```python
from build123d import *

# Parameters (mm, degrees)
F1_DEPTH = 50
F2_R     = 3
F3_DEPTH = 10


with BuildPart() as f1:
    # F0 (on Front) → F1 (new body)
    with BuildSketch(Plane.XZ):
        Polygon((-25, 2.796772), (-25, -15.488228), (25, -15.488228), (0, 2.796772), align=None)
    extrude(amount=F1_DEPTH)

    # F2 (on face) → F3 (join)
    with BuildSketch(Plane.XY.offset(2.796772)):
        with Locations((-13.586, -13.45)):
            Circle(F2_R)
        with Locations((-13.156, -36.55)):
            Circle(F2_R)
    extrude(amount=F3_DEPTH)


with BuildPart() as f4_1:
    # F4: instance of F1
    add(f1.part.mirror(Plane.YZ))


solid = f4_1.part
```
Design review of the part built by this model. Coordinates are the model's own, in mm. A direction names the side the tool comes from. Coordinates: 2 decimals unless noted, no trailing zeros. Loops run counter-clockwise (first coordinate to the right, second up) from the corner with the lowest first, then second, coordinate; pieces in that order, holes last. Notation, with made-up numbers: (-22, 80.25) -> (11, 80.25) arc R26 cw to (11, 111.25) -> close; hole circle Ø11 at (18.25, 10.25). An arc over 180 degrees is marked (long way). Answer as a JSON object with one key per item and string values.
Q1. Tool access review of faces 1 (the flat face through (-12.67, -24.65, -6.47)), 2 (the cylindrical face through (10.295, -35.649, 7.727)): name each direction out of +Z, -Z, +X, -X, +Y, -Y from which nothing blocks a thin tool from reaching the whole face with its end or side.
Answer block:
{"face 1": "+Z, -X, +Y, -Y", "face 2": "+Z"}
Q2. To check wall thickness, follow L1, parallel to Z at x = 6, y = -14; L2, parallel to Z at x = -9, y = -45.5; L3, parallel to X at y = -24, z = -9. State the ranges of each line that lie inside material, in increasing order.
Answer block:
{"L1": "z = -15.49 to 2.8", "L2": "z = -15.49 to -3.79", "L3": "x = -16.13 to 25"}
Q3. Take a section at B-B on y = -13.45. Give the boundary of the cut face in (x, z), plus the area to 3 significant figures.
Answer block:
{"outline": "(-25, -15.49) -> (25, -15.49) -> (25, 2.8) -> (16.59, 2.8) -> (16.59, 12.8) -> (10.59, 12.8) -> (10.59, 2.8) -> (0, 2.8) -> close", "area": "746 mm^2"}
Q4. Take a section at C-C on x = 14. Give the boundary of the cut face in (y, z).
Answer block:
{"outline": "(-50, -15.49) -> (0, -15.49) -> (0, 2.8) -> (-10.48, 2.8) -> (-10.48, 12.8) -> (-16.42, 12.8) -> (-16.42, 2.8) -> (-33.67, 2.8) -> (-33.67, 12.8) -> (-39.43, 12.8) -> (-39.43, 2.8) -> (-50, 2.8) -> close"}
Q5. Clearance check with flat-ended pins moving along their axes: pin 1 Ø1 at (x, y) = (6.5, -38.5) entering from +Z; pin 2 Ø2 at (y, z) = (-17, -10) entering from -X; pin 3 Ø8 at (x, z) = (2, 8.5) entering from -Y. State where each tip first meets the part, or that it passes through.
Answer block:
{"pin 1": "stops at z = 2.8", "pin 2": "stops at x = -18.86", "pin 3": "passes through"}
Q6. Take a section at D-D on y = -5.5. Give the boundary of the cut face in (x, z).
Answer block:
{"outline": "(-25, -15.49) -> (25, -15.49) -> (25, 2.8) -> (0, 2.8) -> close"}
Q7. The part is to be moulded in two halves that separate along Y. For faces 3 (the cylindrical face through (13.977, -10.476, 7.727)), 4 (the flat face through (6, -50, -6)), 5 (the flat face through (13, -37, 12.797)), say which applies: +Y half, -Y half, draft (parallel to the pull), parting line (faces both ways), or undercut.
Answer block:
{"face 3": "undercut", "face 4": "-Y half", "face 5": "draft"}
Q8. Take a section at A-A on z = 6.5. Give the boundary of the cut face in (x, y), plus the area to 3 significant figures.
Answer block:
{"outline": "circle Ø6 at (13.16, -36.55); circle Ø6 at (13.59, -13.45)", "area": "56.5 mm^2"}
